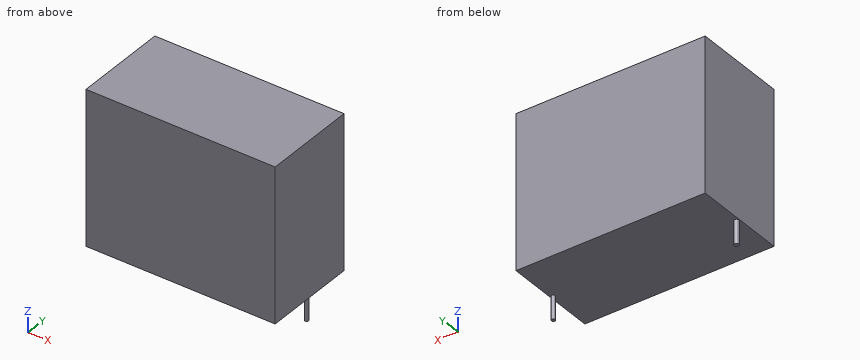
```python
from build123d import *

# Parameters (mm, degrees)
SKETCH_2_W      = 32
SKETCH_2_H      = 16
EXTRUDE_1_DEPTH = 26
SKETCH_3_R      = 0.4
SKETCH_3_R_2    = 0.3
EXTRUDE_2_DEPTH = 4


with BuildPart() as part:
    # Эскиз2 → Вытянуть1 (new body)
    with BuildSketch(Plane.XY):
        with Locations((15.5, 0)):
            Rectangle(SKETCH_2_W, SKETCH_2_H)
    extrude(amount=EXTRUDE_1_DEPTH)

    # Эскиз3 → Вытянуть2 (add)
    with BuildSketch(Plane(origin=(0, 0, 0), x_dir=(-1, 0, 0), z_dir=(0, 0, -1))):
        with Locations(Location((0, 0, 0), (0, 0, 180))):
            Circle(SKETCH_3_R)
        with Locations(Location((-31, 0, 0), (0, 0, 180))):
            Circle(SKETCH_3_R_2)
    extrude(amount=EXTRUDE_2_DEPTH)


solid = part.part
```
Source: CAD feature listing. Evaluate the final solid. Frame: model axes, mm. Coordinates: 2 decimals unless noted, no trailing zeros. Write each loop counter-clockwise with the first axis right and the second up, starting at its lowest first coordinate (ties: lowest second). Pieces come first, ordered by that corner, then holes. Notation, with made-up numbers: (75.5, 9) -> (93.5, 9) arc R25 cw to (93.5, 29) -> close; hole circle Ø5 at (-9, 28). An arc over 180 degrees is marked (long way). Return JSON: item names as keys, results as strings. Group by question number.
1) Contact query for a flat-ended pin moving along its axis: P1, Ø8, axis at x = 14.5, y = 2.5, coming from the -Z side. Output: stop coordinate, or through.
2) Ray query, line 1 along Z through (x, y) = (25, -5.5). Return the intervals inside material, ascending.
3) Section query A-A, the plane x = 0. Return loops of the section in (y, z), plus the area to 3 significant figures.
4) Section query C-C, the plane x = 6. Return loops of the section in (y, z).
5) Section query B-B, the plane y = -5.75. Return loops of the section in (x, z), plus the area to 3 significant figures.
From the geometry:
{
 "1": {"P1": "z = 0"},
 "2": {"line 1": "0 to 26"},
 "3": {"outline": "(-8, 0) -> (-0.4, 0) -> (-0.4, -4) -> (0.4, -4) -> (0.4, 0) -> (8, 0) -> (8, 26) -> (-8, 26) -> close", "area": "419 mm²"},
 "4": {"outline": "(-8, 0) -> (8, 0) -> (8, 26) -> (-8, 26) -> close"},
 "5": {"outline": "(-0.5, 0) -> (31.5, 0) -> (31.5, 26) -> (-0.5, 26) -> close", "area": "832 mm²"}
}
